For this review, take the finished solid that the model builds, in its own axes (mm). A direction names the side the tool comes from. Coordinates: 2 decimals unless noted, no trailing zeros. Order: outer loops, then holes, each group sorted by start corner. A loop starts at its lowest first (then second) coordinate and runs counter-clockwise, first axis right, second up.
Autodesk Inventor part; units mm, degrees
ref_plane "YZ Plane" through (0, 0, 0) normal (1, 0, 0) x (0, 1, 0)
ref_plane "XZ Plane" through (0, 0, 0) normal (0, 1, 0) x (-1, 0, 0)
ref_plane "XY Plane" through (0, 0, 0) normal (0, 0, 1) x (1, 0, 0)
sketch "Sketch1" plane through (0, 0, 0) normal (0, 0, 1) x (1, 0, 0)
  line L0 (-17.78, 6.35) -> (7.62, 6.35)
  line L1 (7.62, 6.35) -> (7.62, -5.715)
  line L2 (7.62, -5.715) -> (-17.78, -5.715)
  line L3 (-17.78, -5.715) -> (-17.78, 6.35)
  point P0 (0, 0)
  dimension "d0" = 25.4
  dimension "d1" = 12.065
  dimension "d2" = 7.62
  dimension "d3" = 6.35
extrude "Extrusion1" add sketch "Sketch1" along normal blind 7.62
sketch "Sketch2" plane through (7.62, -5.715, 0) normal (1, 0, 0) x (0, 0, -1)
  line L0 (-6.35, 10.795) -> (-1.27, 10.795)
  line L1 (-1.27, 10.795) -> (-1.27, 1.27)
  line L2 (-1.27, 1.27) -> (-6.35, 1.27)
  line L3 (-6.35, 1.27) -> (-6.35, 10.795)
  line L4 (-7.62, 0) -> (-7.62, 12.065)
  line L5 (0, 12.065) -> (-7.62, 12.065)
  line L6 (0, 12.065) -> (0, 0)
  line L7 (0, 0) -> (-7.62, 0)
  point P0 (0, 5.715)
  dimension "d8" = 1.27
  dimension "d9" = 1.27
  dimension "d23" = 1.27
  dimension "d24" = 1.27
extrude "Extrusion2" cut sketch "Sketch2" against normal blind 21.59 contours L0 L1 L2 L3
sketch "Sketch3" plane through (0, 0, 7.62) normal (0, 0, 1) x (1, 0, 0)
  line L0 (-17.78, 6.35) -> (-17.78, -5.715)
  line L1 (7.62, 6.35) -> (-17.78, 6.35)
  line L2 (-17.78, -5.715) -> (7.62, -5.715)
  line L3 (-17.78, 6.35) -> (-11.43, 6.35)
  line L4 (-11.43, 6.35) -> (-11.43, -5.715)
  line L5 (-11.43, -5.715) -> (-17.78, -5.715)
  line L6 (-17.78, -5.715) -> (-17.78, 6.35)
  point P0 (0, 0)
  dimension "d26" = 6.35
extrude "Extrusion3" add sketch "Sketch3" along normal blind 25.4
sketch "Sketch4" plane through (0, 0, 7.62) normal (0, 0, 1) x (1, 0, 0)
  circle A0 centre (2.54, -0.635) radius 0.635
  line L0 (7.62, 6.35) -> (-17.78, 6.35)
  point P0 (0, 0)
  point P1 (-11.43, 6.35)
  dimension "d18" = 1.27
  dimension "d20" = 6.985
  dimension "d25" = 2.54
extrude "Extrusion4" cut sketch "Sketch4" against normal blind 50.8
properties part number "hollowPart"
1. Take a section at B-B, the plane x = -3.25. Give the boundary of the cut face in (y, z) (3 decimals), plus the area to 3 significant figures.
Answer below:
outline: (-5.715, 0) - (6.35, 0) - (6.35, 7.62) - (-5.715, 7.62) - close; hole (-4.445, 1.27) - (5.08, 1.27) - (5.08, 6.35) - (-4.445, 6.35) - close
area: 43.5 mm2
2. To check wall thickness, follow L1, parallel to Z at x = 4.25, y = -1.25; L2, parallel to Y at x = 2.54, z = 6.7 (3 decimals); L3, parallel to Z at x = -12, y = 1.25. State the ranges of each line that lie inside material, in increasing order.
Answer below:
L1: z = 0 to 1.27, 6.35 to 7.62
L2: y = -5.715 to -1.27, 0 to 6.35
L3: z = 0 to 1.27, 6.35 to 33.02
3. Machinability: for faces 5 (the face through (7.62, 0, 1)), 6 (the face through (-3, 5.08, 4)), 7 (the face through (-2, 0, 7.62)), which of the approach directions +Z, -Z, +X, -X, +Y, -Y give a long, thin tool a straight path to every point of the face, cutting with its end or side? Answer none if there is none.
Answer below:
face 5: +Z, -Z, +X, +Y, -Y
face 6: +X
face 7: +Z, +X, +Y, -Y
4. Take a section at A-A, the plane x = 2.54. Give the boundary of the cut face in (y, z) (3 decimals).
Answer below:
outline: (-5.715, 0) - (-1.27, 0) - (-1.27, 1.27) - (-4.445, 1.27) - (-4.445, 6.35) - (-1.27, 6.35) - (-1.27, 7.62) - (-5.715, 7.62) - close; (0, 0) - (6.35, 0) - (6.35, 7.62) - (0, 7.62) - (0, 6.35) - (5.08, 6.35) - (5.08, 1.27) - (0, 1.27) - close
5. Take a section at D-D, the plane z = 5. Give the boundary of the cut face in (x, y) (3 decimals).
Answer below:
outline: (-17.78, -5.715) - (7.62, -5.715) - (7.62, -4.445) - (-13.97, -4.445) - (-13.97, 5.08) - (7.62, 5.08) - (7.62, 6.35) - (-17.78, 6.35) - close
6. Take a section at C-C, the plane y = -4. Give the boundary of the cut face in (x, z).
Answer below:
outline: (-17.78, 0) - (7.62, 0) - (7.62, 1.27) - (-13.97, 1.27) - (-13.97, 6.35) - (7.62, 6.35) - (7.62, 7.62) - (-11.43, 7.62) - (-11.43, 33.02) - (-17.78, 33.02) - close
7. Clearance check with flat-ended pins moving along their axes: pin 1 Ø1.1 at (x, y) = (2.54, -0.635) entering from -Z; pin 2 Ø5 at (x, y) = (-7, -1) entering from +Z; pin 3 Ø1.5 at (y, z) = (-2, 4) entering from +X; pin 4 Ø6 at (y, z) = (0.5, 21) entering from +X. State where each tip first meets the part, or that it passes through.
Answer below:
pin 1: passes through
pin 2: stops at z = 7.62
pin 3: stops at x = -13.97
pin 4: stops at x = -11.43
8. The part is to be moulded in two halves that separate along Y. For faces 1 (the face through (-13, 6.35, 9)), 2 (the face through (-17.78, 0, 16)), 3 (the face through (-3, 0, 1.27)), 4 (the face through (-14, -5.715, 9)), say which applies: +Y half, -Y half, draft (parallel to the pull), parting line (faces both ways), or undercut.
Answer below:
face 1: +Y half
face 2: draft
face 3: undercut
face 4: -Y half
